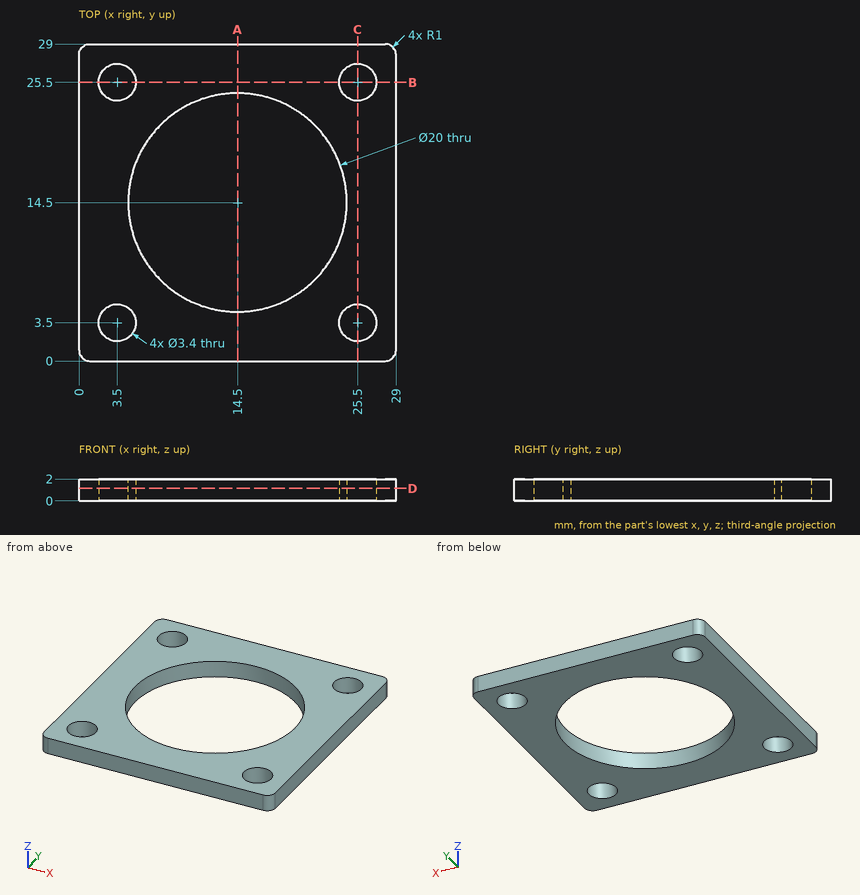
Part print with two shaded views. Sizes in mm from the minimum x, y, z corner. Give positions to 0.01 mm unless a question says otherwise; leave off trailing zeros. Order: outer loops, then holes, each group sorted by start corner. A loop starts at its lowest first (then second) coordinate and runs counter-clockwise, first axis right, second up.
(1) Saw through at A-A, the plane x = 14.5. Give the cut face in (y, z), then the cut area to 3 significant figures.
(2) Saw through at D-D, the plane z = 1.15. Give the cut face in (x, y), then the cut area to 3 significant figures.
(3) Saw through at B-B, the plane y = 25.5. Give the cut face in (x, z).
(4) Drill centre lines: L1, parallel to Y at x = 14.5, z = 1.6; L2, parallel to Y at x = 25.5, z = 1.5; L3, parallel to X at y = 27, z = 0.2. Where is each one in solid material? Low to high.
Results found:
1. outline: (0, 0) - (4.5, 0) - (4.5, 2) - (0, 2) - close; (24.5, 0) - (29, 0) - (29, 2) - (24.5, 2) - close
1. area: 18.0 mm2
2. outline: (0, 1) arc R1 ccw to (1, 0) - (28, 0) arc R1 ccw to (29, 1) - (29, 28) arc R1 ccw to (28, 29) - (1, 29) arc R1 ccw to (0, 28) - close; hole circle Ø3.4 at (3.5, 3.5); hole circle Ø3.4 at (3.5, 25.5); hole circle Ø20 at (14.5, 14.5); hole circle Ø3.4 at (25.5, 3.5); hole circle Ø3.4 at (25.5, 25.5)
2. area: 490 mm2
3. outline: (0, 0) - (1.8, 0) - (1.8, 2) - (0, 2) - close; (5.2, 0) - (23.8, 0) - (23.8, 2) - (5.2, 2) - close; (27.2, 0) - (29, 0) - (29, 2) - (27.2, 2) - close
4. L1: y = 0 to 4.5, 24.5 to 29
4. L2: y = 0 to 1.8, 5.2 to 23.8, 27.2 to 29
4. L3: x = 0 to 2.7, 4.3 to 24.7, 26.3 to 29
